Part model, mm, in its own coordinate system. Give positions to 0.01 mm unless a question says otherwise; leave off trailing zeros. Order: outer loops, then holes, each group sorted by start corner. A loop starts at its lowest first (then second) coordinate and runs counter-clockwise, first axis right, second up. Notation, with made-up numbers: (30, 70) - (86, 70) arc R26 cw to (86, 88) - close; hole circle Ø6 at (77.25, -12.75). An arc over 180 degrees is marked (long way). One line per item, written item: value.
```python
from build123d import *

# Parameters (mm, degrees)
SKETCH1_W               = 19.05
SKETCH1_H               = 19.05
SKETCH1_W_2             = 15.875
SKETCH1_H_2             = 15.875
BOSS_EXTRUDE1_DEPTH     = 609.6
CUT_EXTRUDE1_DEPTH      = 610.748809962
CUT_EXTRUDE1_DEPTH_BACK = 610.748809962
SKETCH2_R               = 3.175
SKETCH3_R               = 3.175
CUT_EXTRUDE2_DEPTH      = 610.971956835


with BuildPart() as part:
    # Sketch1 → Boss-Extrude1 (new, symmetric)
    with BuildSketch(Plane.XY):
        Rectangle(SKETCH1_W, SKETCH1_H)
        Rectangle(SKETCH1_W_2, SKETCH1_H_2, mode=Mode.SUBTRACT)
    extrude(amount=BOSS_EXTRUDE1_DEPTH, both=True)

    # Sketch2 → Cut-Extrude1 (cut, two sides: drawn at the far end of the back side and taken through both)
    with BuildSketch(Plane(origin=(0, 0, 0), x_dir=(1, 0, 0), z_dir=(0, 1, 0)).offset(-CUT_EXTRUDE1_DEPTH_BACK)):
        with Locations(Location((0, -596.9, 0), (0, 0, 270))):
            Circle(SKETCH2_R)
        with Locations(Location((0, -571.5, 0), (0, 0, 270))):
            Circle(SKETCH2_R)
        with Locations(Location((0, -444.5, 0), (0, 0, 270))):
            Circle(SKETCH2_R)
        with Locations(Location((0, -419.1, 0), (0, 0, 270))):
            Circle(SKETCH2_R)
        with Locations(Location((0, -292.1, 0), (0, 0, 270))):
            Circle(SKETCH2_R)
        with Locations(Location((0, -266.7, 0), (0, 0, 270))):
            Circle(SKETCH2_R)
    extrude(amount=CUT_EXTRUDE1_DEPTH + CUT_EXTRUDE1_DEPTH_BACK, mode=Mode.SUBTRACT)

    # Sketch3 → Cut-Extrude2 (cut, through all)
    with BuildSketch(Plane.ZY.offset(9.525)):
        with Locations((-152.4, 0)):
            Circle(SKETCH3_R)
        with Locations((73.03, 0)):
            Circle(SKETCH3_R)
    extrude(amount=-CUT_EXTRUDE2_DEPTH, mode=Mode.SUBTRACT)


solid = part.part
```
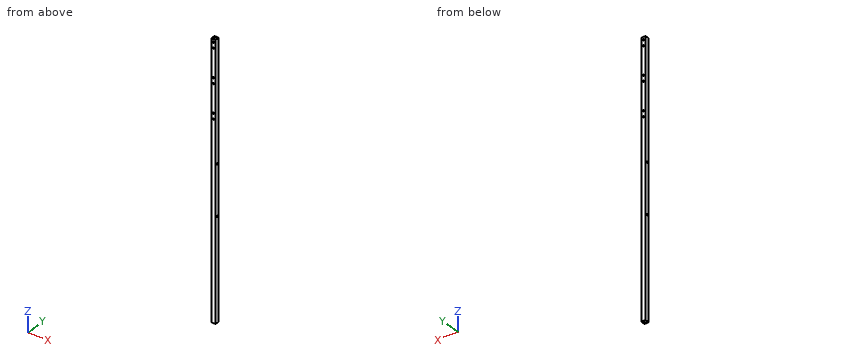
1) Slice it at A-A on y = 0. Write the cut outline in (x, z) (1 decimal).
Answer:
outline: (-9.5, -609.6) - (-7.9, -609.6) - (-7.9, -155.6) - (-9.5, -155.6) - close; (-9.5, -149.2) - (-7.9, -149.2) - (-7.9, 69.9) - (-9.5, 69.9) - close; (-9.5, 76.2) - (-7.9, 76.2) - (-7.9, 609.6) - (-9.5, 609.6) - close; (7.9, -609.6) - (9.5, -609.6) - (9.5, -155.6) - (7.9, -155.6) - close; (7.9, -149.2) - (9.5, -149.2) - (9.5, 69.9) - (7.9, 69.9) - close; (7.9, 76.2) - (9.5, 76.2) - (9.5, 609.6) - (7.9, 609.6) - close
2) Drop a flat-ended pin along its axis: P1, Ø4, axis at x = 0, z = 419.1, coming from the +Y side. Give the stop position or say it passes through.
Answer:
P1: passes through
3) Slice it at B-B on z = -235.5. Write the cut outline in (x, y) (1 decimal), then the cut area to 3 significant figures.
Answer:
outline: (-9.5, -9.5) - (9.5, -9.5) - (9.5, 9.5) - (-9.5, 9.5) - close; hole (-7.9, -7.9) - (7.9, -7.9) - (7.9, 7.9) - (-7.9, 7.9) - close
area: 111 mm2
4) Wall check: line 1 along Y through (x, z) = (5.75, 19) (1 decimal); line 2 along Y through (x, z) = (8.3, -152.4) (3 decimals). Give the ranges that are in metal, low to high. Write a range as [from, to].
Answer:
line 1: y = [-9.5, -7.9], [7.9, 9.5]
line 2: y = [-9.525, -3.175], [3.175, 9.525]
5) Slice it at C-C on x = 0. Count the separate pieces of the cut face and the enclosed holes in it, then the cut area to 3 significant figures.
Answer:
separate pieces: 14
enclosed holes: 0
area: 3,750 mm2
